Verification items for the finished model (mm, model axes). A direction names the side the tool comes from. Round coordinates to 2 decimals unless told otherwise and drop trailing zeros. Loops run counter-clockwise (first coordinate to the right, second up) from the corner with the lowest first, then second, coordinate; pieces in that order, holes last. Notation, with made-up numbers: (66.5, -17.5) - (88.5, -17.5) arc R24 ccw to (88.5, 9.5) - close; hole circle Ø4 at (85, 4). An arc over 180 degrees is marked (long way). Use CSV: the item, a comma, the result in double quotes.
```python
from build123d import *

# Parameters (mm, degrees)
F0_W     = 38.1
F0_H     = 38.1
F1_DEPTH = 38.1
F6_DEPTH = 38.1
F8_DEPTH = 38.1


with BuildPart() as f1:
    # F0 (on Front) → F1 (new body)
    with BuildSketch(Plane.XZ):
        with Locations((19.05, 19.05)):
            Rectangle(F0_W, F0_H)
    extrude(amount=F1_DEPTH)

    # F5 (on offset) → F6 (cut)
    with BuildSketch(Plane.XZ.offset(38.1)):
        Polygon((31.75, 38.1), (6.35, 38.1), (11.43, 15.875), (16.51, 28.575), (21.59, 28.575), (26.67, 15.875), align=None)
        Polygon((0, 0), (6.35, 0), (0, 38.1), align=None)
        Polygon((19.05, 15.875), (12.7, 0), (25.4, 0), align=None)
        Polygon((38.1, 38.1), (31.75, 0), (38.1, 0), align=None)
    extrude(amount=-F6_DEPTH, mode=Mode.SUBTRACT)

    # F7 (on offset) → F8 (cut)
    with BuildSketch(Plane.YZ.offset(38.1)):
        Polygon((-26.67, 22.225), (-31.75, 0), (-6.35, 0), (-11.43, 22.225), (-16.51, 9.525), (-21.59, 9.525), align=None)
        Polygon((-31.75, 38.1), (-38.1, 38.1), (-38.1, 0), align=None)
        Polygon((-6.35, 38.1), (0, 0), (0, 38.1), align=None)
        Polygon((-12.7, 38.1), (-25.4, 38.1), (-19.05, 22.225), align=None)
    extrude(amount=-F8_DEPTH, mode=Mode.SUBTRACT)


solid = f1.part
```
1) Gauge pin test, flat ends, axial feed: pin 1 Ø6 at (y, z) = (-33.5, 27) entering from +X; pin 2 Ø5.5 at (x, y) = (13, -18.5) entering from -Z (3 decimals); pin 3 Ø1.5 at (y, z) = (-32.5, 25.5) entering from -X (3 decimals). Record the tip position at first contact, or that the pin passes through.
Returned:
pin 1,"stops at x = 36.75"
pin 2,"stops at z = 9.525"
pin 3,"stops at x = 1.975"
2) Access from +Z, -Z, +X, -X, +Y, -Y to the whole of each face (thin tool, end or side, straight path). Record for faces 4 (the face through (15.9, -5.1, 8)), 5 (the face through (19, -28, 28.575)), 6 (the face through (11, -19, 9.525)), 7 (the face through (29, -35, 0)), 8 (the face through (33.2, -15.9, 30.1)).
Returned:
face 4,"-Z, +Y, -Y"
face 5,"+Z, +Y, -Y"
face 6,"-Z, +X, -X"
face 7,"-Z, +X, -X, +Y, -Y"
face 8,"+Z, +X, -X"
3) Cross-section at A-A, the plane z = 33. Record the cut outline in (x, y).
Returned:
outline,"(0.85, -32.6) - (7.52, -32.6) - (7.52, -23.36) - (0.85, -23.36) - close; (0.85, -14.74) - (7.52, -14.74) - (7.52, -5.5) - (0.85, -5.5) - close; (30.58, -32.6) - (37.25, -32.6) - (37.25, -23.36) - (30.58, -23.36) - close; (30.58, -14.74) - (37.25, -14.74) - (37.25, -5.5) - (30.58, -5.5) - close"
4) Cross-section at B-B, the plane y = -27.5. Count the separate pieces of the cut face and the enclosed holes in it, then the cut area to 3 significant figures.
Returned:
separate pieces,"3"
enclosed holes,"0"
area,"362 mm²"
5) Mould release check, pull along Y, two halves, no side actions. Record for faces 1 (the face through (19, -11, 28.575)), 2 (the face through (28, -19, 9.525)), 3 (the face through (19.32, -34.97, 18.78)): +Y half, -Y half, draft (parallel to the pull), parting line (faces both ways), or undercut.
Returned:
face 1,"draft"
face 2,"undercut"
face 3,"-Y half"
6) Cross-section at C-C, the plane z = 11. Record the cut outline in (x, y).
Returned:
outline,"(4.52, -36.27) - (17.1, -36.27) - (17.1, -29.24) - (4.52, -29.24) - close; (4.52, -22.18) - (17.1, -22.18) - (17.1, -15.92) - (4.52, -15.92) - close; (4.52, -8.86) - (17.1, -8.86) - (17.1, -1.83) - (4.52, -1.83) - close; (21, -36.27) - (33.58, -36.27) - (33.58, -29.24) - (21, -29.24) - close; (21, -22.18) - (33.58, -22.18) - (33.58, -15.92) - (21, -15.92) - close; (21, -8.86) - (33.58, -8.86) - (33.58, -1.83) - (21, -1.83) - close"
7) Thickness scan on probe 1 along Y at (x, z) = (26.5, 13); probe 2 along X at (y, z) = (-5, 24); probe 3 along Y at (x, z) = (33, 11). Record the ranges inside material, lowest first. Write a range as [from, to].
Returned:
probe 1,"y = [-35.93, -28.78], [-22.98, -15.12], [-9.32, -2.17]"
probe 2,"x = [2.35, 9.57], [14.68, 23.42], [28.53, 35.75]"
probe 3,"y = [-36.27, -29.24], [-22.18, -15.92], [-8.86, -1.83]"
